Check sheet for the modelled part. Datum: model origin and axes. Units: mm. Face numbers are marked on the shaded views. A direction names the side the tool comes from. Coordinates: 2 decimals unless noted, no trailing zeros. Loops run counter-clockwise (first coordinate to the right, second up) from the corner with the lowest first, then second, coordinate; pieces in that order, holes last. Notation, with made-up numbers: M 37,18 L 72,18 A20 ccw 72,45 Z; hole C 77,18.25 d8. An arc over 180 degrees is marked long. Write each question's results on one line, items separated by ' | '. Start each with the question number.
from build123d import *

# Parameters (mm, degrees)
SKETCH_1_W          = 40
SKETCH_1_H          = 30
EXTRUDE_1_DEPTH     = 5
SKETCH_2_W          = 31
SKETCH_2_H          = 28
CUT_EXTRUDE_1_DEPTH = 3.5
CUT_EXTRUDE_2_DEPTH = 26.243811123
EXTRUDE_START       = 8
EXTRUDE_2_DEPTH     = 8
FILLET_START        = 1.5
FILLET_1_DEPTH      = 8.5
CHAMFER_1_SIZE      = 3
EXTRUDE_3_DEPTH     = 5
SKETCH_7_W          = 7
SKETCH_7_H          = 3
EXTRUDE_4_DEPTH     = 1.5


with BuildPart() as part:
    # ｽｹｯﾁ1 → ﾎﾞｽ - 押し出し1 (new body)
    with BuildSketch(Plane.XY):
        Rectangle(SKETCH_1_W, SKETCH_1_H)
    extrude(amount=EXTRUDE_1_DEPTH)

    # ｽｹｯﾁ2 → ｶｯﾄ - 押し出し1 (cut)
    with BuildSketch(Plane.XY.offset(5)):
        with Locations((0, -1)):
            Rectangle(SKETCH_2_W, SKETCH_2_H)
    extrude(amount=-CUT_EXTRUDE_1_DEPTH, mode=Mode.SUBTRACT)

    # ｽｹｯﾁ3 → ｶｯﾄ - 押し出し2 (cut, through all)
    with BuildSketch(Plane.XY.offset(1.5)):
        with BuildLine():
            Line((8.5, -2), (8.5, -15))
            Line((8.5, -15), (-8.5, -15))
            Line((-8.5, -15), (-8.5, -2))
            ThreePointArc((-8.5, -2), (0, 6.5), (8.5, -2))
        make_face()
        with BuildLine():
            Line((13, -4.5), (13, 0.5))
            ThreePointArc((13, 0.5), (11.5, 2), (10, 0.5))
            Line((10, 0.5), (10, -4.5))
            ThreePointArc((10, -4.5), (11.5, -6), (13, -4.5))
        make_face()
        with BuildLine():
            Line((-13, -4.5), (-13, 0.5))
            ThreePointArc((-13, 0.5), (-11.5, 2), (-10, 0.5))
            Line((-10, 0.5), (-10, -4.5))
            ThreePointArc((-10, -4.5), (-11.5, -6), (-13, -4.5))
        make_face()
    extrude(amount=-CUT_EXTRUDE_2_DEPTH, mode=Mode.SUBTRACT)

    # ｽｹｯﾁ4 → ﾎﾞｽ - 押し出し2 (add)
    with BuildSketch(Plane.XY.offset(1.5).offset(EXTRUDE_START)):
        with BuildLine():
            Line((-8.5, -2), (-8.5, 13))
            Line((-8.5, 13), (8.5, 13))
            Line((8.5, 13), (8.5, -2))
            ThreePointArc((8.5, -2), (0, 6.5), (-8.5, -2))
        make_face()
    extrude(amount=-EXTRUDE_2_DEPTH)

    # ﾌｨﾚｯﾄ1: read off the stored shape, not the designer's step
    # ﾌｨﾚｯﾄ1 outline → ﾌｨﾚｯﾄ1 (cut)
    with BuildSketch(Plane.XY.offset(FILLET_START)):
        with BuildLine():
            ThreePointArc((8.5, 2.123105626), (8.117851131, 1.637192968), (7.555555556, 1.894044202))
            ThreePointArc((7.555555556, 1.894044202), (8.260515184, 0.003469213), (8.5, -2))
            Line((8.5, -2), (8.5, 2.123105626))
        make_face()
        with BuildLine():
            ThreePointArc((-7.555555556, 1.894044202), (-8.117851131, 1.637192968), (-8.5, 2.123105626))
            Line((-8.5, 2.123105626), (-8.5, -2))
            ThreePointArc((-8.5, -2), (-8.260515184, 0.003469213), (-7.555555556, 1.894044202))
        make_face()
    extrude(amount=FILLET_1_DEPTH, mode=Mode.SUBTRACT)

    # 面取り1
    chamfer_1_edges = [part.edges().sort_by_distance(p)[0] for p in [
        (0, 13, 9.5),
    ]]
    chamfer(chamfer_1_edges, length=CHAMFER_1_SIZE)

    # ｽｹｯﾁ5 → ﾎﾞｽ - 押し出し3 (add)
    with BuildSketch(Plane(origin=(0, 0, 0), x_dir=(-1, 0, 0), z_dir=(0, 0, -1))):
        Polygon((-15.5, -15), (-20, -15), (-20, -20), (20, -20), (20, -15), (15.5, -15), (15.5, -18), (8.5, -18), (-8.5, -18), (-15.5, -18), align=None)
    extrude(amount=-EXTRUDE_3_DEPTH)

    # ｽｹｯﾁ7 → ﾎﾞｽ - 押し出し4 (add)
    with BuildSketch(Plane(origin=(0, 0, 0), x_dir=(-1, 0, 0), z_dir=(0, 0, -1))):
        with Locations((12, -16.5)):
            Rectangle(SKETCH_7_W, SKETCH_7_H)
        with Locations((-12, -16.5)):
            Rectangle(SKETCH_7_W, SKETCH_7_H)
    extrude(amount=-EXTRUDE_4_DEPTH)


solid = part.part
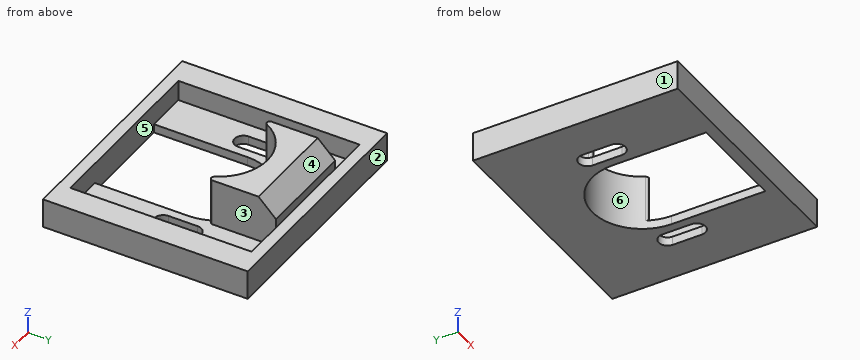
Item 1: Thickness scan on line 1 (X direction, y = -4, z = 1.25); line 2 (X direction, y = -16, z = 4); line 3 (X direction, y = -15.5, z = 1). Record the ranges inside material, lowest first.
Item 2: Section check D-D (y = 1). Record the cut outline in (x, z), plus the area to 3 significant figures.
Item 3: Release check for a two-part mould opening along X. For the marked faces 1, 2 and 3 record: +X half, -X half, draft (parallel to the pull), parting line (faces both ways), or undercut.
Item 4: Depth check by flat-ended pin: P1, Ø1.5, axis at y = -10, z = 7.5, coming from the +X side; P2, Ø10.5, axis at x = 5.5, y = 3, coming from the +Z side; P3, Ø2.5, axis at x = -11, y = 5, coming from the +Z side. Enter the tip coordinate at first touch or a pass-through.
Item 5: Tool access check on the marked faces 4, 5 and 6. Record the directions out of +Z, -Z, +X, -X, +Y, -Y that give a thin tool (end or side, any length) a straight path to the whole face; none if there is none.
Item 6: Section check B-B (x = 0). Record the cut outline in (y, z), plus the area to 4 significant figures.
Item 7: Section check A-A (y = -10.5). Record the cut outline in (x, z), plus the area to 3 significant figures.
Item 8: Section check C-C (x = 9). Record the cut outline in (y, z).
Computed values:
1) line 1: x = -20 to -13, -10 to -8.5, 8.5 to 10, 13 to 20 | line 2: x = -20 to -15.5, 15.5 to 20 | line 3: x = -20 to -8.5, 8.5 to 20
2) outline: M -20,0 L -12.91,0 L -12.91,1.5 L -15.5,1.5 L -15.5,5 L -20,5 Z; M -10.09,0 L -7.95,0 L -7.95,1.5 L -10.09,1.5 Z; M 7.95,0 L 10.09,0 L 10.09,1.5 L 7.95,1.5 Z; M 12.91,0 L 20,0 L 20,5 L 15.5,5 L 15.5,1.5 L 12.91,1.5 Z | area: 59.2 mm²
3) face 1: -X half | face 2: draft | face 3: undercut
4) P1: passes through | P2: stops at z = 9.5 | P3: stops at z = 1.5
5) face 4: +Z, +X, -X, +Y | face 5: +Z | face 6: +Z, -Z
6) outline: M -20,0 L -18,0 L -18,5 L -20,5 Z; M 6.5,0 L 15,0 L 15,5 L 13,5 L 13,6.5 L 10,9.5 L 6.5,9.5 Z | area: 77.25 mm²
7) outline: M -20,0 L -8.5,0 L -8.5,1.5 L -15.5,1.5 L -15.5,5 L -20,5 Z; M 8.5,0 L 20,0 L 20,5 L 15.5,5 L 15.5,1.5 L 8.5,1.5 Z | area: 66.0 mm²
8) outline: M -20,0 L 15,0 L 15,5 L 13,5 L 13,1.5 L -18,1.5 L -18,5 L -20,5 Z
